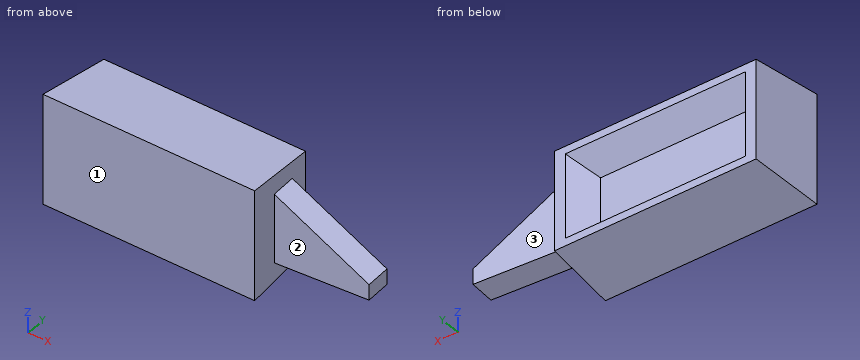
from build123d import *

# Parameters (mm, degrees)
SKETCH1_W           = 205.785682804
SKETCH1_H           = 104.534748446
BOSS_EXTRUDE1_DEPTH = 70.104
BOSS_EXTRUDE1_TAPER = 4
SKETCH2_W           = 145.758865666
SKETCH2_H           = 50.974097726
CUT_EXTRUDE1_DEPTH  = 25.4
SKETCH3_W           = 65.29816474
SKETCH3_H           = 24.799651417
BOSS_EXTRUDE2_DEPTH = 87.63
DRAFT1_ANGLE        = 30
DRAFT2_ANGLE        = 30


with BuildPart() as part:
    # Sketch1 → Boss-Extrude1 (new body)
    with BuildSketch(Plane(origin=(0, 0, 0), x_dir=(1, 0, 0), z_dir=(0, 1, 0))):
        Rectangle(SKETCH1_W, SKETCH1_H)
    extrude(amount=BOSS_EXTRUDE1_DEPTH, taper=BOSS_EXTRUDE1_TAPER)

    # Sketch2 → Cut-Extrude1 (cut)
    with BuildSketch(Plane(origin=(0, 70.104, 0), x_dir=(1, 0, 0), z_dir=(0, 1, 0))):
        Rectangle(SKETCH2_W, SKETCH2_H)
    extrude(amount=-CUT_EXTRUDE1_DEPTH, mode=Mode.SUBTRACT)

    # Sketch3 → Boss-Extrude2 (add)
    with BuildSketch(Plane(origin=(102.392168372, 7.159957902, 0), x_dir=(0, 0, -1), z_dir=(0.9975640502598242, 0.06975647374412534, 0))):
        with Locations((0, 32.321763147)):
            Rectangle(SKETCH3_W, SKETCH3_H)
    extrude(amount=BOSS_EXTRUDE2_DEPTH)

    # Draft1
    draft1_faces = [part.faces().sort_by_distance(p)[0] for p in [
        (0, 57.404, 25.487048863),
        (72.879432833, 57.404, 0),
        (0, 57.404, -25.487048863),
        (-72.879432833, 57.404, 0),
    ]]
    draft(draft1_faces, Plane.ZX.offset(44.704), DRAFT1_ANGLE)

    # Draft2
    draft2_faces = [part.faces().sort_by_distance(p)[0] for p in [
        (143.845785012, 42.459366756, 32.64908237),
    ]]
    draft(draft2_faces, Plane(origin=(102.892841402, 0, 52.267374223), x_dir=(-0.06975647374412534, 0.9975640502598243, 0), z_dir=(0.9975640502598243, 0.06975647374412534, 0)), DRAFT2_ANGLE)


solid = part.part
Verification items for the finished model (mm, model axes). Face numbers are marked on the shaded views. Give positions to 0.01 mm unless a question says otherwise; leave off trailing zeros. Write each loop counter-clockwise with the first axis right and the second up, starting at its lowest first coordinate (ties: lowest second). Pieces come first, ordered by that corner, then holes. Notation, with made-up numbers: (46.25, -31.5) - (55.25, -31.5) arc R20 ccw to (55.25, -7.5) - close; hole circle Ø7 at (-29.75, -10). An arc over 180 degrees is marked (long way). Answer as CSV lines item,"result". Start each with the question number.
1. Sectioned sample at A-A (x = 160). Record the boundary of the cut face in (y, z).
2. Thickness scan on line 1 (Y direction, x = -42, z = -2.5); line 2 (Z direction, x = 0, y = 61.5); line 3 (X direction, y = 50, z = -9). Record the ranges inside material, lowest first.
3. Draft check along X on the marked faces 1, 2 and 3. Enter one of: pulls with the +X half, pulls with the -X half, needs draft (parallel to the pull), parting line crosses it, or undercut.
4. Depth check by flat-ended pin: pin 1 (5 mm diameter, centred on y = 22.5, z = 7.5, fed in from +X); pin 2 (1 mm diameter, centred on x = 5, z = -2.5, fed in from +Y); pin 3 (1.5 mm diameter, centred on x = 5.5, z = -37, fed in from -Y); pin 4 (12 mm diameter, centred on x = -5, y = 41.5, fed in from -Z) (3 decimals). Enter the tip coordinate at first touch or a pass-through.
Derived:
1,outline,"(31.16, -32.65) - (56.02, -32.65) - (56.02, -2.5) - (31.16, -1.5) - close"
2,line 1,"0 to 44.7"
2,line 2,"-47.97 to -35.18, 35.18 to 47.97"
2,line 3,"-99.4 to -75.94, 75.94 to 171.71"
3,face 1,"needs draft"
3,face 2,"pulls with the +X half"
3,face 3,"undercut"
4,pin 1,"x = 101.49"
4,pin 2,"y = 44.7"
4,pin 3,"y = 0"
4,pin 4,"z = -49.785"
